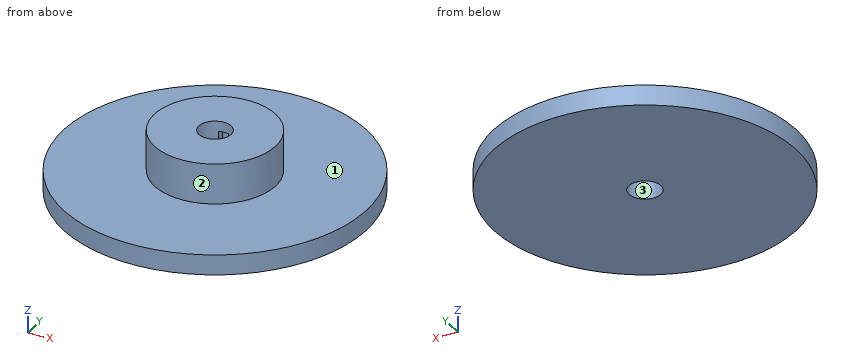
from build123d import *

# Parameters (mm, degrees)
SKETCH1_R           = 75
BOSS_EXTRUDE1_DEPTH = 10
SKETCH2_R           = 30
BOSS_EXTRUDE2_DEPTH = 20
SKETCH3_R           = 8
CUT_EXTRUDE1_DEPTH  = 111.227038425
CUT_EXTRUDE2_START  = -5
SKETCH4_W           = 5
SKETCH4_H           = 6
CUT_EXTRUDE2_DEPTH  = 20


with BuildPart() as part:
    # Sketch1 → Boss-Extrude1 (new body)
    with BuildSketch(Plane.XY):
        Circle(SKETCH1_R)
    extrude(amount=BOSS_EXTRUDE1_DEPTH)

    # Sketch2 → Boss-Extrude2 (add)
    with BuildSketch(Plane.XY.offset(10)):
        Circle(SKETCH2_R)
    extrude(amount=BOSS_EXTRUDE2_DEPTH)

    # Sketch3 → Cut-Extrude1 (cut, through all)
    with BuildSketch(Plane.XY.offset(30)):
        Circle(SKETCH3_R)
    extrude(amount=-CUT_EXTRUDE1_DEPTH, mode=Mode.SUBTRACT)

    # Sketch4 → Cut-Extrude2 (cut)
    with BuildSketch(Plane.XY.offset(30).offset(CUT_EXTRUDE2_START)):
        with Locations((0, 8)):
            Rectangle(SKETCH4_W, SKETCH4_H)
    extrude(amount=-CUT_EXTRUDE2_DEPTH, mode=Mode.SUBTRACT)


solid = part.part
Geometry check sheet. Reference: the model listing, model coordinates, mm. Face numbers are marked on the shaded views. Give positions to 0.01 mm unless a question says otherwise; leave off trailing zeros. Order: outer loops, then holes, each group sorted by start corner. A loop starts at its lowest first (then second) coordinate and runs counter-clockwise, first axis right, second up.
1. Sectioned sample at B-B (x = 0). Record the boundary of the cut face in (y, z), then the cut area to 3 significant figures.
Completed:
outline: (-75, 0) - (-8, 0) - (-8, 30) - (-30, 30) - (-30, 10) - (-75, 10) - close; (8, 0) - (75, 0) - (75, 10) - (30, 10) - (30, 30) - (8, 30) - (8, 25) - (11, 25) - (11, 5) - (8, 5) - close
area: 2,160 mm2
2. Draft check along X on the marked faces 1, 2 and 3. Enter one of: pulls with the +X half, pulls with the -X half, needs draft (parallel to the pull), parting line crosses it, or undercut.
Completed:
face 1: needs draft
face 2: parting line crosses it
face 3: undercut
3. Sectioned sample at C-C (x = -18.5). Record the boundary of the cut face in (y, z).
Completed:
outline: (-72.68, 0) - (72.68, 0) - (72.68, 10) - (23.62, 10) - (23.62, 30) - (-23.62, 30) - (-23.62, 10) - (-72.68, 10) - close
4. Scan lines: line 1 (Y direction, x = 0, z = 10.25); line 2 (Y direction, x = 0, z = 7); line 3 (Z direction, x = -65, y = -25.5). Record each from-to range of solid material in increasing order.
Completed:
line 1: y = -30 to -8, 11 to 30
line 2: y = -75 to -8, 11 to 75
line 3: z = 0 to 10
5. Depth check by flat-ended pin: pin 1 (1.5 mm diameter, centred on x = -0.5, z = 11.5, fed in from -Y); pin 2 (1.5 mm diameter, centred on x = -10, z = 20.5, fed in from -Y); pin 3 (1 mm diameter, centred on y = 8.5, z = 18, fed in from -X). Enter the tip coordinate at first touch or a pass-through.
Completed:
pin 1: stops at y = -30
pin 2: stops at y = -28.54
pin 3: stops at x = -28.91
6. Sectioned sample at A-A (y = 0). Record the boundary of the cut face in (x, z), then the cut area to 3 significant figures.
Completed:
outline: (-75, 0) - (-8, 0) - (-8, 30) - (-30, 30) - (-30, 10) - (-75, 10) - close; (8, 0) - (75, 0) - (75, 10) - (30, 10) - (30, 30) - (8, 30) - close
area: 2,220 mm2
7. Sectioned sample at D-D (y = -52). Record the boundary of the cut face in (x, z), then the cut area to 3 significant figures.
Completed:
outline: (-54.05, 0) - (54.05, 0) - (54.05, 10) - (-54.05, 10) - close
area: 1,080 mm2
